from build123d import *

# Parameters (mm, degrees)
SKETCH1_R           = 5
SKETCH1_R_2         = 1.7
BOSS_EXTRUDE1_DEPTH = 10
SKETCH1_4_R         = 5
SKETCH1_4_R_2       = 1.7
CUT_EXTRUDE1_DEPTH  = 4
SKETCH3_W           = 6
SKETCH3_H           = 1.0375
SKETCH3_W_2         = 2
BOSS_EXTRUDE2_DEPTH = 10
BOSS_EXTRUDE3_DEPTH = 5
SKETCH3_4_W         = 2
SKETCH3_4_H         = 10
SKETCH3_4_W_2       = 6
SKETCH3_4_H_2       = 1.0375
BOSS_EXTRUDE4_DEPTH = 2


with BuildPart() as part:
    # Sketch1 → Boss-Extrude1 (new body)
    # profile 1 of 4: a face of its own
    with BuildSketch(Plane.XY):
        with BuildLine():
            Line((-48, 22.22), (-48, 20))
            ThreePointArc((-48, 20), (-42.142135624, 5.857864376), (-28, 0))
            Line((-28, 0), (0, 0))
            Line((0, 0), (0, 10))
            Line((0, 10), (-18, 10))
            ThreePointArc((-18, 10), (-25.071067812, 12.928932188), (-28, 20))
            Line((-28, 20), (-28, 22.22))
            ThreePointArc((-28, 22.22), (-38, 32.22), (-48, 22.22))
        make_face()
        with Locations((-38, 22.22)):
            Circle(SKETCH1_R, mode=Mode.SUBTRACT)
    # profile 2 of 4: a face of its own
    with BuildSketch(Plane.XY):
        with Locations((-38, 22.22)):
            Circle(SKETCH1_R)
        with Locations((-38, 22.22)):
            Circle(SKETCH1_R_2, mode=Mode.SUBTRACT)
    # profile 3 of 4: a face of its own
    with BuildSketch(Plane.XY):
        with BuildLine():
            Line((0, 10), (0, 0))
            Line((0, 0), (28, 0))
            ThreePointArc((28, 0), (42.142135624, 5.857864376), (48, 20))
            Line((48, 20), (48, 22.22))
            ThreePointArc((48, 22.22), (38, 32.22), (28, 22.22))
            Line((28, 22.22), (28, 20))
            ThreePointArc((28, 20), (25.071067812, 12.928932188), (18, 10))
            Line((18, 10), (0, 10))
        make_face()
        with Locations((38, 22.22)):
            Circle(SKETCH1_R, mode=Mode.SUBTRACT)
    # profile 4 of 4: a face of its own
    with BuildSketch(Plane.XY):
        with Locations((38, 22.22)):
            Circle(SKETCH1_R)
        with Locations((38, 22.22)):
            Circle(SKETCH1_R_2, mode=Mode.SUBTRACT)
    extrude(amount=-BOSS_EXTRUDE1_DEPTH)

    # Sketch1<4> → Cut-Extrude1 (cut)
    # profile 1 of 2: a face of its own
    with BuildSketch(Plane.XY):
        with Locations((-38, 22.22)):
            Circle(SKETCH1_4_R)
        with Locations((-38, 22.22)):
            Circle(SKETCH1_4_R_2, mode=Mode.SUBTRACT)
    # profile 2 of 2: a face of its own
    with BuildSketch(Plane.XY):
        with Locations((38, 22.22)):
            Circle(SKETCH1_4_R)
        with Locations((38, 22.22)):
            Circle(SKETCH1_4_R_2, mode=Mode.SUBTRACT)
    extrude(amount=-CUT_EXTRUDE1_DEPTH, mode=Mode.SUBTRACT)

    # Sketch3 → Boss-Extrude2 (add, through all)
    with BuildSketch(Plane.XY):
        with Locations((-3, 10.51875)):
            Rectangle(SKETCH3_W, SKETCH3_H)
        with Locations((3, 10.51875)):
            Rectangle(SKETCH3_W, SKETCH3_H)
        with Locations((-3, -0.51875)):
            Rectangle(SKETCH3_W, SKETCH3_H)
        with Locations((3, -0.51875)):
            Rectangle(SKETCH3_W, SKETCH3_H)
        with Locations((-7, 10.51875)):
            Rectangle(SKETCH3_W_2, SKETCH3_H)
        Polygon((-15, 10), (-8, 10), (-8, 11.0375), (-8, 11.5375), (-15, 11.5375), align=None)
        Polygon((-8, 11.0375), (-6, 11.0375), (-6, 13.5375), (-15, 13.5375), (-15, 11.5375), (-8, 11.5375), align=None)
        Polygon((-6, -3.5375), (-6, -1.0375), (-8, -1.0375), (-8, -1.5375), (-15, -1.5375), (-15, -3.5375), align=None)
        with Locations((-7, -0.51875)):
            Rectangle(SKETCH3_W_2, SKETCH3_H)
        with Locations((7, -0.51875)):
            Rectangle(SKETCH3_W_2, SKETCH3_H)
        Polygon((8, -1.0375), (6, -1.0375), (6, -3.5375), (15, -3.5375), (15, -1.5375), (8, -1.5375), align=None)
        Polygon((8, 0), (8, -1.0375), (8, -1.5375), (15, -1.5375), (15, 0), align=None)
        Polygon((8, 11.0375), (8, 10), (15, 10), (15, 11.5375), (8, 11.5375), align=None)
        with Locations((7, 10.51875)):
            Rectangle(SKETCH3_W_2, SKETCH3_H)
        Polygon((6, 13.5375), (6, 11.0375), (8, 11.0375), (8, 11.5375), (15, 11.5375), (15, 13.5375), align=None)
        Polygon((-8, -1.5375), (-8, -1.0375), (-8, 0), (-15, 0), (-15, -1.5375), align=None)
    extrude(amount=-BOSS_EXTRUDE2_DEPTH)

    # Sketch3<3> → Boss-Extrude3 (add)
    with BuildSketch(Plane.XY):
        Polygon((-8, 11.0375), (-6, 11.0375), (-6, 13.5375), (-15, 13.5375), (-15, 11.5375), (-8, 11.5375), align=None)
        Polygon((-6, -3.5375), (-6, -1.0375), (-8, -1.0375), (-8, -1.5375), (-15, -1.5375), (-15, -3.5375), align=None)
        Polygon((8, -1.0375), (6, -1.0375), (6, -3.5375), (15, -3.5375), (15, -1.5375), (8, -1.5375), align=None)
        Polygon((6, 13.5375), (6, 11.0375), (8, 11.0375), (8, 11.5375), (15, 11.5375), (15, 13.5375), align=None)
    extrude(amount=BOSS_EXTRUDE3_DEPTH)

    # Sketch3<4> → Boss-Extrude4 (add)
    with BuildSketch(Plane.XY):
        with Locations((-7, 5)):
            Rectangle(SKETCH3_4_W, SKETCH3_4_H)
        with Locations((-3, 5)):
            Rectangle(SKETCH3_4_W_2, SKETCH3_4_H)
        with Locations((7, 5)):
            Rectangle(SKETCH3_4_W, SKETCH3_4_H)
        with Locations((3, 5)):
            Rectangle(SKETCH3_4_W_2, SKETCH3_4_H)
        with Locations((3, 10.51875)):
            Rectangle(SKETCH3_4_W_2, SKETCH3_4_H_2)
        with Locations((7, 10.51875)):
            Rectangle(SKETCH3_4_W, SKETCH3_4_H_2)
        with Locations((-3, 10.51875)):
            Rectangle(SKETCH3_4_W_2, SKETCH3_4_H_2)
        with Locations((-7, 10.51875)):
            Rectangle(SKETCH3_4_W, SKETCH3_4_H_2)
        with Locations((-7, -0.51875)):
            Rectangle(SKETCH3_4_W, SKETCH3_4_H_2)
        with Locations((-3, -0.51875)):
            Rectangle(SKETCH3_4_W_2, SKETCH3_4_H_2)
        with Locations((3, -0.51875)):
            Rectangle(SKETCH3_4_W_2, SKETCH3_4_H_2)
        with Locations((7, -0.51875)):
            Rectangle(SKETCH3_4_W, SKETCH3_4_H_2)
    extrude(amount=BOSS_EXTRUDE4_DEPTH)


solid = part.part
Geometry: final body of the model. Coordinates: model frame, mm. A direction names the side the tool comes from. Give positions to 0.01 mm unless a question says otherwise; leave off trailing zeros. Write each loop counter-clockwise with the first axis right and the second up, starting at its lowest first coordinate (ties: lowest second). Pieces come first, ordered by that corner, then holes.
(1) Mould query, pull axis Y, two halves, no side actions, for faces 6 (the flat face through (10, -3.538, -2)), 7 (the flat face through (12, -1.538, 2)), 8 (the flat face through (10, -3, 5)). Classes: released by +Y, released by -Y, zero draft, split by the parting line, or undercut.
(2) Cut plane B-B, the plane x = 38. Return loops of the section in (y, z).
(3) Cut plane A-A, the plane z = -8.5. Give the number of separate pieces and of enclosed holes in the cut face, then the cut area to 3 significant figures.
(4) Ray query, line 1 (X direction, y = 22, z = -5.75); line 2 (Z direction, x = -7, y = 4); line 3 (Z direction, x = -34.5, y = 11). Return the intervals inside material, ascending.
(5) Cut plane D-D, the plane y = 15.5. Return loops of the section in (x, z), then the cut area to 3 significant figures.
(6) Cut plane C-C, the plane z = 3.5. Return loops of the section in (x, y).
(7) Access query for faces 1 (the flat face through (-15, -2, -4)), 2 (the flat face through (0, 5, 2)), 3 (the flat face through (-8, 5, 1)), 4 (the flat face through (11, 11.538, 2)), 5 (the flat face through (6, 12, -2)). Directions: +Z, -Z, +X, -X, +Y, -Y. A direction counts if a zero-diameter tool reaches every point of the face in a straight line with its end or side. Return the directions, or none.
(8) First-contact query: P1, Ø4, axis at y = 9, z = -1, coming from the +X side; P2, Ø6, axis at x = -36, y = 16.5, coming from the +Z side; P3, Ø2.5, axis at x = 8.5, z = -2.5, coming from the +Y side; P4, Ø2, axis at x = -38, y = 22.22, coming from the -Z side. Flat tips, straight axial feed; report the tip coordinate or a pass-through.
Values follow:
1. face 6: released by -Y
1. face 7: undercut
1. face 8: zero draft
2. outline: (2.68, -10) - (20.52, -10) - (20.52, -4) - (17.22, -4) - (17.22, 0) - (2.68, 0) - close; (23.92, -10) - (32.22, -10) - (32.22, 0) - (27.22, 0) - (27.22, -4) - (23.92, -4) - close
3. separate pieces: 1
3. enclosed holes: 2
3. area: 1,770 mm2
4. line 1: x = -48 to -39.69, -36.31 to -28, 28 to 36.31, 39.69 to 48
4. line 2: z = -10 to 2
4. line 3: z = -10 to 0
5. outline: (-47.49, -10) - (-26.93, -10) - (-26.93, 0) - (-47.49, 0) - close; (26.93, -10) - (47.49, -10) - (47.49, 0) - (26.93, 0) - close
5. area: 411 mm2
6. outline: (-15, -3.54) - (-6, -3.54) - (-6, -1.04) - (-8, -1.04) - (-8, -1.54) - (-15, -1.54) - close; (-15, 11.54) - (-8, 11.54) - (-8, 11.04) - (-6, 11.04) - (-6, 13.54) - (-15, 13.54) - close; (6, -3.54) - (15, -3.54) - (15, -1.54) - (8, -1.54) - (8, -1.04) - (6, -1.04) - close; (6, 11.04) - (8, 11.04) - (8, 11.54) - (15, 11.54) - (15, 13.54) - (6, 13.54) - close
7. face 1: +Z, -Z, -X, -Y
7. face 2: +Z, +X, -X
7. face 3: +Z, -X
7. face 4: +Z, +X
7. face 5: +Z, -Z, +Y
8. P1: stops at x = 45.86
8. P2: stops at z = 0
8. P3: stops at y = 13.54
8. P4: passes through
